Geometry check sheet. Reference: the model listing, model coordinates, mm. Face numbers are marked on the shaded views. A direction names the side the tool comes from. Coordinates: 2 decimals unless noted, no trailing zeros. Loops run counter-clockwise (first coordinate to the right, second up) from the corner with the lowest first, then second, coordinate; pieces in that order, holes last. Notation, with made-up numbers: (45.25, -26) - (61.25, -26) arc R8 ccw to (61.25, -17) - close; hole circle Ø10 at (73.5, -11.75). An arc over 180 degrees is marked (long way). One line per item, written item: value.
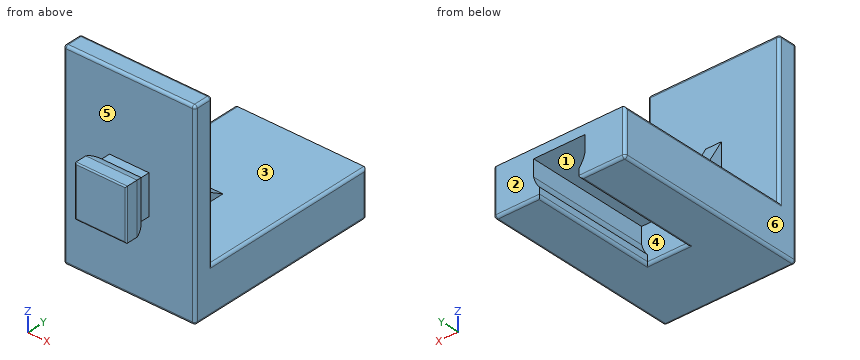
from build123d import *

# Parameters (mm, degrees)
EXTRUDE_1_DEPTH      = 5
EXTRUDE_1_DEPTH_BACK = 5
EXTRUDE_2_DEPTH      = 0.6
EXTRUDE_2_DEPTH_BACK = 0.6
SKETCH_3_W           = 3
SKETCH_3_H           = 3
EXTRUDE_3_DEPTH      = 1
EXTRUDE_4_DEPTH      = 1
EXTRUDE_4_DEPTH_BACK = 4
CUT_EXTRUDE_1_REACH  = 20.154
CUT_EXTRUDE_2_DEPTH  = 9.45
FILLET_1_R           = 0.1
FILLET_2_R           = 0.2


with BuildPart() as part:
    # 草图1 → 凸台-拉伸1 (new, two sides: drawn at the far end of the back side and taken through both)
    with BuildSketch(Plane(origin=(0, 0, 0), x_dir=(0, 0, -1), z_dir=(1, 0, 0)).offset(-EXTRUDE_1_DEPTH_BACK)):
        Polygon((-7.5, 0), (7.5, 0), (7.5, 15), (4, 15), (4, 1.5), (-7.5, 1.5), align=None)
    extrude(amount=EXTRUDE_1_DEPTH + EXTRUDE_1_DEPTH_BACK)

    # 草图2 → 凸台-拉伸2 (add, two sides: drawn at the far end of the back side and taken through both)
    with BuildSketch(Plane(origin=(0, 0, 0), x_dir=(0, 0, -1), z_dir=(1, 0, 0)).offset(-EXTRUDE_2_DEPTH_BACK)):
        Polygon((-2, 1.5), (1.803847577, 3.696152423), (4, 7.5), (4, 1.5), align=None)
    extrude(amount=EXTRUDE_2_DEPTH + EXTRUDE_2_DEPTH_BACK)

    # 草图3 → 凸台-拉伸3 (add)
    with BuildSketch(Plane.XZ):
        Rectangle(SKETCH_3_W, SKETCH_3_H)
    extrude(amount=EXTRUDE_3_DEPTH)

    # 草图4 → 凸台-拉伸4 (add, two sides: drawn at the far end of the back side and taken through both)
    with BuildSketch(Plane.XY.offset(1.5).offset(-EXTRUDE_4_DEPTH_BACK)):
        with BuildLine():
            Line((-1.95, -2.5), (1.95, -2.5))
            Line((1.95, -2.5), (1.95, -1.555590279))
            ThreePointArc((1.95, -1.555590279), (1.780042303, -1.088161527), (1.5, -0.677124344))
            Line((1.5, -0.677124344), (-1.5, -0.677124344))
            ThreePointArc((-1.5, -0.677124344), (-1.780042303, -1.088161527), (-1.95, -1.555590279))
            Line((-1.95, -1.555590279), (-1.95, -2.5))
        make_face()
    extrude(amount=EXTRUDE_4_DEPTH + EXTRUDE_4_DEPTH_BACK)

    # 草图5 → 切除-拉伸1 (cut, up to next)
    with BuildSketch(Plane.ZY.offset(1.95), mode=Mode.PRIVATE) as cut_extrude_1_sk1:
        with BuildLine():
            Line((-1.95, -2.5), (-1.95, -1.555590279))
            ThreePointArc((-1.95, -1.555590279), (-1.780042303, -1.088161527), (-1.5, -0.677124344))
            Line((-1.5, -0.677124344), (-2.5, -0.677124344))
            Line((-2.5, -0.677124344), (-2.5, -2.5))
            Line((-2.5, -2.5), (-1.95, -2.5))
        make_face()
    cut_extrude_1_tool1 = extrude(cut_extrude_1_sk1.sketch, amount=-CUT_EXTRUDE_1_REACH, mode=Mode.PRIVATE) & part.part
    # 草图5 → 切除-拉伸1 (cut, up to next)
    with BuildSketch(Plane.ZY.offset(1.95), mode=Mode.PRIVATE) as cut_extrude_1_sk2:
        with BuildLine():
            Line((2.5, -2.5), (2.5, -0.677124344))
            Line((2.5, -0.677124344), (1.5, -0.677124344))
            ThreePointArc((1.5, -0.677124344), (1.780042303, -1.088161527), (1.95, -1.555590279))
            Line((1.95, -1.555590279), (1.95, -2.5))
            Line((1.95, -2.5), (2.5, -2.5))
        make_face()
    cut_extrude_1_tool2 = extrude(cut_extrude_1_sk2.sketch, amount=-CUT_EXTRUDE_1_REACH, mode=Mode.PRIVATE) & part.part
    add(cut_extrude_1_tool1.solids().sort_by_distance((-1.95, -1.500125, -2.169375))[0], mode=Mode.SUBTRACT)
    add(cut_extrude_1_tool2.solids().sort_by_distance((-1.95, -1.500125, 2.169375))[0], mode=Mode.SUBTRACT)

    # 草图6 → 切除-拉伸2 (cut)
    with BuildSketch(Plane(origin=(0, 15, 0), x_dir=(-1, 0, 0), z_dir=(0, 1, 0))):
        with BuildLine():
            Line((1.5, -7.5), (-1.5, -7.5))
            Line((-1.5, -7.5), (-1.5, -6.822875656))
            ThreePointArc((-1.5, -6.822875656), (-1.780042303, -6.411838473), (-1.95, -5.944409721))
            Line((-1.95, -5.944409721), (-1.95, -4.7))
            Line((-1.95, -4.7), (1.95, -4.7))
            Line((1.95, -4.7), (1.95, -5.944409721))
            ThreePointArc((1.95, -5.944409721), (1.780042303, -6.411838473), (1.5, -6.822875656))
            Line((1.5, -6.822875656), (1.5, -7.5))
        make_face()
    extrude(amount=-CUT_EXTRUDE_2_DEPTH, mode=Mode.SUBTRACT)

    # 圆角1
    fillet_1_edges = [part.edges().sort_by_distance(p)[0] for p in [
        (-1.95, -2.5, 0),
        (1.95, -2.5, 0),
        (0, -2.5, -1.95),
        (0, -2.5, 1.95),
    ]]
    fillet(fillet_1_edges, radius=FILLET_1_R)

    # 圆角2
    fillet_2_edges = [part.edges().sort_by_distance(p)[0] for p in [
        (-5, 7.5, -7.5),
        (0, 1.5, 7.5),
        (-3.25, 15, -7.5),
        (0, 0, -7.5),
        (0, 0, 7.5),
        (3.25, 15, -7.5),
        (0, 5.55, -7.5),
        (-1.5, 10.275, -7.5),
        (1.5, 10.275, -7.5),
        (-5, 15, -5.75),
        (-5, 8.25, -4),
        (5, 0.75, 7.5),
        (5, 0, 0),
        (5, 7.5, -7.5),
        (5, 15, -5.75),
        (5, 8.25, -4),
        (-5, 1.5, 1.75),
        (5, 1.5, 1.75),
        (-5, 0.75, 7.5),
        (-5, 0, 0),
    ]]
    fillet(fillet_2_edges, radius=FILLET_2_R)


solid = part.part
(1) Release check for a two-part mould opening along X. For the marked faces 4, 5 and 6 record: pulls with the +X half, pulls with the -X half, needs draft (parallel to the pull), parting line crosses it, or undercut.
Reply:
face 4: undercut
face 5: needs draft
face 6: pulls with the -X half
(2) Cross-section at D-D on z = 6.5. Record the cut outline in (x, y).
Reply:
outline: (-5, 0.2) arc R0.2 ccw to (-4.8, 0) - (4.8, 0) arc R0.2 ccw to (5, 0.2) - (5, 1.3) arc R0.2 ccw to (4.8, 1.5) - (-4.8, 1.5) arc R0.2 ccw to (-5, 1.3) - close
(3) Go/stop test with flat-tipped pins: pin 1 Ø0.7 at (y, z) = (-2, -0.5) entering from +X; pin 2 Ø5 at (x, z) = (1, -3) entering from -Y; pin 3 Ø1.2 at (x, y) = (0, 11) entering from -Z. Record where each tip stops, or that it passes through.
Reply:
pin 1: x = 1.95
pin 2: y = -2.5
pin 3: z = -4.7
(4) Cross-section at B-B on y = 10.5. Record the cut outline in (x, z), and give its area (3 significant figures).
Reply:
outline: (-5, -7.3) arc R0.2 ccw to (-4.8, -7.5) - (-1.7, -7.5) arc R0.2 ccw to (-1.5, -7.3) - (-1.5, -6.82) arc R2 cw to (-1.95, -5.94) - (-1.95, -4.7) - (1.95, -4.7) - (1.95, -5.94) arc R2 cw to (1.5, -6.82) - (1.5, -7.3) arc R0.2 ccw to (1.7, -7.5) - (4.8, -7.5) arc R0.2 ccw to (5, -7.3) - (5, -4.2) arc R0.2 ccw to (4.8, -4) - (-4.8, -4) arc R0.2 ccw to (-5, -4.2) - close
area: 25.0 mm2
(5) Material ranges on probe 1 along Z at (x, y) = (3.5, 13); probe 2 along Y at (x, z) = (-2.25, 3); probe 3 along X at (y, z) = (9, -5.75), recorded low to high. Write a range as from..to.
Reply:
probe 1: -7.5..-4
probe 2: 0..1.5
probe 3: -5..-1.95, 1.95..5
(6) Cross-section at C-C on x = 3. Record the cut outline in (y, z).
Reply:
outline: (0, -7.3) arc R0.2 ccw to (0.2, -7.5) - (14.8, -7.5) arc R0.2 ccw to (15, -7.3) - (15, -4) - (1.5, -4) - (1.5, 7.3) arc R0.2 ccw to (1.3, 7.5) - (0.2, 7.5) arc R0.2 ccw to (0, 7.3) - close
(7) Cross-section at A-A on z = -5.5. Record the cut outline in (x, y).
Reply:
outline: (-5, 0.2) arc R0.2 ccw to (-4.8, 0) - (4.8, 0) arc R0.2 ccw to (5, 0.2) - (5, 14.8) arc R0.2 ccw to (4.8, 15) - (1.95, 15) - (1.95, 5.55) - (-1.95, 5.55) - (-1.95, 15) - (-4.8, 15) arc R0.2 ccw to (-5, 14.8) - close
(8) Access from +Z, -Z, +X, -X, +Y, -Y to the whole of each face (thin tool, end or side, straight path). Record for the marked faces 1, 2 and 3.
Reply:
face 1: +Y
face 2: +Z, -Z, +X, -X, +Y
face 3: +Z, +Y
